```python
from build123d import *

# Parameters (mm, degrees)
SKETCH1_W           = 18
SKETCH1_H           = 5
SKETCH1_W_2         = 2
SKETCH1_H_2         = 2
SKETCH1_H_3         = 50
BOSS_EXTRUDE1_DEPTH = 35
SKETCH2_W           = 2.9
SKETCH2_H           = 45
BOSS_EXTRUDE2_DEPTH = 5
SKETCH3_W           = 6
SKETCH3_H           = 30.514407746
CUT_EXTRUDE1_DEPTH  = 5


with BuildPart() as part:
    # Sketch1 → Boss-Extrude1 (new body)
    with BuildSketch(Plane.XY):
        with Locations((23.3, 4.5)):
            Rectangle(SKETCH1_W, SKETCH1_H)
        Polygon((2, 2), (2, 0), (32.3, 0), (32.3, 2), (14.3, 2), align=None)
        with Locations((1, 1)):
            Rectangle(SKETCH1_W_2, SKETCH1_H_2)
        with Locations((1, 27)):
            Rectangle(SKETCH1_W_2, SKETCH1_H_3)
    extrude(amount=BOSS_EXTRUDE1_DEPTH)

    # Sketch2 → Boss-Extrude2 (add)
    with BuildSketch(Plane(origin=(2, 0, 0), x_dir=(0, 0, -1), z_dir=(1, 0, 0))):
        with Locations((-33.55, 29.5)):
            Rectangle(SKETCH2_W, SKETCH2_H)
        with Locations((-1.45, 29.5)):
            Rectangle(SKETCH2_W, SKETCH2_H)
    extrude(amount=BOSS_EXTRUDE2_DEPTH)

    # Sketch3 → Cut-Extrude1 (cut)
    with BuildSketch(Plane.XZ):
        with Locations((5, 17.5)):
            Rectangle(SKETCH3_W, SKETCH3_H)
    extrude(amount=-CUT_EXTRUDE1_DEPTH, mode=Mode.SUBTRACT)


solid = part.part
```
The listing builds one solid part. Answer for the finished solid, in the listing's coordinates (mm). A direction names the side the tool comes from. Round coordinates to 2 decimals unless told otherwise and drop trailing zeros. Write each loop counter-clockwise with the first axis right and the second up, starting at its lowest first coordinate (ties: lowest second). Pieces come first, ordered by that corner, then holes. Notation, with made-up numbers: (0, 64.25) -> (10, 64.25) arc R25 ccw to (10, 81.25) -> close; hole circle Ø8 at (46, 39). An arc over 180 degrees is marked (long way). Write item = value, one per line.
1) For a pull along Z with two mould halves and no side action, classify faces 1 (the flat face through (6.5, 24.2, 0)), 2 (the flat face through (5, 1, 2.243)), 3 (the flat face through (4, 29, 2.9)), 4 (the flat face through (16, 0, 17)) as released by +Z, released by -Z, zero draft, split by the parting line, or undercut.
Check values:
face_1 = released by -Z
face_2 = undercut
face_3 = undercut
face_4 = zero draft
2) Section B-B on z = 8.5 is taken. Write down the section's boundary in (x, y), plus the area to 3 significant figures.
Check values:
outline = (0, 0) -> (2, 0) -> (2, 52) -> (0, 52) -> close; (8, 0) -> (32.3, 0) -> (32.3, 7) -> (14.3, 7) -> (14.3, 2) -> (8, 2) -> close
area = 243 mm²
3) Section D-D on y = 16 is taken. Write down the section's boundary in (x, z).
Check values:
outline = (0, 0) -> (7, 0) -> (7, 2.9) -> (2, 2.9) -> (2, 32.1) -> (7, 32.1) -> (7, 35) -> (0, 35) -> close
4) Which of the six approach directions +Z, -Z, +X, -X, +Y, -Y give full straight-line access (tool end or side, diameter ignored) to faces 5 (the flat face through (7, 30, 34)), 6 (the flat face through (4, 7, 1)), 7 (the flat face through (14.3, 4, 17))?
Check values:
face_5 = +Z, -Z, +X, +Y
face_6 = +Z, -Z
face_7 = +Z, -Z, +Y
5) Straight lines are drawn through the part: line 1 along X through (y, z) = (6, 9); line 2 along X through (y, z) = (50.5, 24); line 3 along Y through (x, z) = (24, 3). For each, find the intervals that lie inside material, in ascending order. Write a range as [from, to].
Check values:
line_1 = [0, 2], [14.3, 32.3]
line_2 = [0, 2]
line_3 = [0, 7]
6) Given pin 1 (2.5 mm diameter, centred on y = 23.5, z = 33.5, fed in from +X); pin 2 (12 mm diameter, centred on y = 35, z = 14.5, fed in from +X); pin 3 (5 mm diameter, centred on x = 19, z = 27, fed in from +Y), each flat-ended and moving along its own axis, determine where each tip first touches the part or whether it passes through.
Check values:
pin_1 = 7
pin_2 = 2
pin_3 = 7
7) Section C-C on x = 11 is taken. Write down the section's boundary in (y, z).
Check values:
outline = (0, 0) -> (2, 0) -> (2, 35) -> (0, 35) -> close
8) Section A-A on y = 4 is taken. Write down the section's boundary in (x, z).
Check values:
outline = (0, 0) -> (2, 0) -> (2, 35) -> (0, 35) -> close; (14.3, 0) -> (32.3, 0) -> (32.3, 35) -> (14.3, 35) -> close
